Check sheet for the modelled part. Datum: model origin and axes. Units: mm. A direction names the side the tool comes from. Round coordinates to 2 decimals unless told otherwise and drop trailing zeros. Order: outer loops, then holes, each group sorted by start corner. A loop starts at its lowest first (then second) coordinate and runs counter-clockwise, first axis right, second up.
(1) Sectioned sample at C-C, the plane z = -43. Enter the section's corners in (x, y), and give its area (3 significant figures).
(2) Thickness scan on probe 1 along Z at (x, y) = (5, 55); probe 2 along Y at (x, z) = (10.5, -46). Record the ranges inside material, lowest first.
(3) Tool access check on faces 4 (the flat face through (12, 56, -2)), 5 (the flat face through (-5, 119, -28)), 6 (the flat face through (19, 119.1, -12)). Record the directions out of +Z, -Z, +X, -X, +Y, -Y that give a thin tool (end or side, any length) a straight path to the whole face; none if there is none.
(4) Sectioned sample at D-D, the plane z = -51. Enter the section's corners in (x, y).
(5) Depth check by flat-ended pin: pin 1 (0.6 mm diameter, centred on y = 54, z = -1, fed in from -X); pin 2 (16.5 mm diameter, centred on x = 19, z = -21, fed in from -Y). Enter the tip coordinate at first touch or a pass-through.
(6) Sectioned sample at A-A, the plane y = 103. Enter the section's corners in (x, z).
(7) Mould release check, pull along Y, two halves, no side actions. Record for faces 1 (the cylindrical face through (13.56, 8, -0.99)), 2 (the flat face through (11, 63, 0)), 3 (the cylindrical face through (4.68, 10.02, -55.01)): released by +Y, released by -Y, zero draft, split by the parting line, or undercut.
(8) Sectioned sample at B-B, the plane z = -28. Enter the section's corners in (x, y).
```python
from build123d import *

# Parameters (mm, degrees)
SKETCH1_W               = 28
SKETCH1_H               = 124.1
BOSS_EXTRUDE1_DEPTH     = 2
CUT_EXTRUDE2_DEPTH      = 1
CUT_EXTRUDE2_DEPTH_BACK = 2
SKETCH4_R               = 1.25
CUT_EXTRUDE3_DEPTH      = 2
CIRPATTERN1_COUNT       = 5
CIRPATTERN1_ANGLE       = 180
FILLET1_R               = 1.5
SKETCH7_W               = 28
SKETCH7_H               = 124.1
BOSS_EXTRUDE2_DEPTH     = 2
CUT_EXTRUDE4_DEPTH      = 1
CUT_EXTRUDE4_DEPTH_BACK = 2
SKETCH11_R              = 1.25
CUT_EXTRUDE5_DEPTH      = 2
CIRPATTERN2_COUNT       = 5
CIRPATTERN2_ANGLE       = 180
FILLET2_R               = 1.5
SKETCH17_W              = 33
SKETCH17_H              = 52
BOSS_EXTRUDE5_DEPTH     = 15
CUT_EXTRUDE7_REACH      = 126.1
SKETCH18_R              = 3.05
SKETCH19_R              = 1.25
CUT_EXTRUDE8_DEPTH      = 10
SKETCH20_W              = 29.100039055
SKETCH20_H              = 52
CUT_EXTRUDE9_DEPTH      = 5
SKETCH21_W              = 5
SKETCH21_H              = 15
BOSS_EXTRUDE6_DEPTH     = 2
SKETCH22_W              = 52
SKETCH22_H              = 5
CUT_EXTRUDE10_DEPTH     = 2.95
SKETCH23_W              = 52
SKETCH23_H              = 5
CUT_EXTRUDE11_DEPTH     = 2.949960945
CUT_EXTRUDE12_DEPTH     = 3
SKETCH25_R              = 2.5
CUT_EXTRUDE13_DEPTH     = 5


with BuildPart() as part:
    # Sketch1 → Boss-Extrude1 (new body)
    with BuildSketch(Plane.XY):
        with Locations((14, 62.05)):
            Rectangle(SKETCH1_W, SKETCH1_H)
    extrude(amount=-BOSS_EXTRUDE1_DEPTH)

    # Sketch3 → Cut-Extrude2 (cut, two sides)
    with BuildSketch(Plane.XY) as cut_extrude2_sk:
        with BuildLine():
            Line((18.449960945, -261.260932316), (18.449960945, 0))
            Line((18.449960945, 0), (18.449960945, 3))
            ThreePointArc((18.449960945, 3), (13.449960945, 8), (8.449960945, 3))
            Line((8.449960945, 3), (8.449960945, 0))
            Line((8.449960945, 0), (8.449960945, -261.260932316))
            Line((8.449960945, -261.260932316), (8.449960945, -783.782796947))
            Line((8.449960945, -783.782796947), (18.449960945, -783.782796947))
            Line((18.449960945, -783.782796947), (18.449960945, -261.260932316))
        make_face()
    extrude(amount=CUT_EXTRUDE2_DEPTH, mode=Mode.SUBTRACT)
    extrude(cut_extrude2_sk.sketch, amount=-CUT_EXTRUDE2_DEPTH_BACK, mode=Mode.SUBTRACT)

    # Sketch4 → Cut-Extrude3 (cut)
    with BuildSketch(Plane.XY):
        with Locations((2.449960945, 3)):
            Circle(SKETCH4_R)
    cut_extrude3 = extrude(amount=-CUT_EXTRUDE3_DEPTH, mode=Mode.SUBTRACT)

    # CirPattern1: Cut-Extrude3 ×5 about axis
    cirpattern1_axis = Axis((13.449960945, 3, 0), (0, 0, -1))
    for i in range(1, CIRPATTERN1_COUNT):
        add(cut_extrude3.rotate(cirpattern1_axis, i * CIRPATTERN1_ANGLE / (CIRPATTERN1_COUNT - 1)), mode=Mode.SUBTRACT)

    # Fillet1
    fillet1_edges = [part.edges().sort_by_distance(p)[0] for p in [
        (18.449960945, 0, -1),
        (8.449960945, 0, -1),
        (28, 0, -1),
        (0, 0, -1),
    ]]
    fillet(fillet1_edges, radius=FILLET1_R)



with BuildPart() as body_2:
    # Sketch7 → Boss-Extrude2 (new body)
    with BuildSketch(Plane.XY.offset(-56)):
        with Locations((14, 62.05)):
            Rectangle(SKETCH7_W, SKETCH7_H)
    extrude(amount=BOSS_EXTRUDE2_DEPTH)

    # Sketch10 → Cut-Extrude4 (cut, two sides)
    with BuildSketch(Plane(origin=(0, 0, -56), x_dir=(-1, 0, 0), z_dir=(0, 0, -1))) as cut_extrude4_sk:
        with BuildLine():
            Line((-8.449960945, -261.260932316), (-8.449960945, 0))
            Line((-8.449960945, 0), (-8.449960945, 3))
            ThreePointArc((-8.449960945, 3), (-13.449960945, 8), (-18.449960945, 3))
            Line((-18.449960945, 3), (-18.449960945, 0))
            Line((-18.449960945, 0), (-18.449960945, -261.260932316))
            Line((-18.449960945, -261.260932316), (-18.449960945, -783.782796947))
            Line((-18.449960945, -783.782796947), (-8.449960945, -783.782796947))
            Line((-8.449960945, -783.782796947), (-8.449960945, -261.260932316))
        make_face()
    extrude(amount=CUT_EXTRUDE4_DEPTH, mode=Mode.SUBTRACT)
    extrude(cut_extrude4_sk.sketch, amount=-CUT_EXTRUDE4_DEPTH_BACK, mode=Mode.SUBTRACT)

    # Sketch11 → Cut-Extrude5 (cut)
    with BuildSketch(Plane(origin=(0, 0, -56), x_dir=(-1, 0, 0), z_dir=(0, 0, -1))):
        with Locations((-24.449960945, 3)):
            Circle(SKETCH11_R)
    cut_extrude5 = extrude(amount=-CUT_EXTRUDE5_DEPTH, mode=Mode.SUBTRACT)

    # CirPattern2: Cut-Extrude5 ×5 about axis
    cirpattern2_axis = Axis((13.449960945, 3, 0), (0, 0, 1))
    for i in range(1, CIRPATTERN2_COUNT):
        add(cut_extrude5.rotate(cirpattern2_axis, i * CIRPATTERN2_ANGLE / (CIRPATTERN2_COUNT - 1)), mode=Mode.SUBTRACT)

    # Fillet2
    fillet2_edges = [body_2.edges().sort_by_distance(p)[0] for p in [
        (8.449960945, 0, -55),
        (18.449960945, 0, -55),
        (28, 0, -55),
        (0, 0, -55),
    ]]
    fillet(fillet2_edges, radius=FILLET2_R)


with BuildPart() as part_1:
    add(part.part)

    add(body_2.part)  # Boss-Extrude5 merges body 2
    # Sketch17 → Boss-Extrude5 (add)
    with BuildSketch(Plane(origin=(0, 124.1, 0), x_dir=(1, 0, 0), z_dir=(0, 1, 0))):
        with Locations((11.5, 28)):
            Rectangle(SKETCH17_W, SKETCH17_H)
    extrude(amount=-BOSS_EXTRUDE5_DEPTH)

    # Sketch18 → Cut-Extrude7 (cut, up to next)
    with BuildSketch(Plane(origin=(0, 124.1, 0), x_dir=(1, 0, 0), z_dir=(0, 1, 0)), mode=Mode.PRIVATE) as cut_extrude7_sk1:
        with Locations((13.449960945, 28)):
            Circle(SKETCH18_R)
    cut_extrude7_tool1 = extrude(cut_extrude7_sk1.sketch, amount=-CUT_EXTRUDE7_REACH, mode=Mode.PRIVATE) & part_1.part
    add(cut_extrude7_tool1.solids().sort_by_distance((13.449961, 124.1, -28))[0], mode=Mode.SUBTRACT)

    # Sketch19 → Cut-Extrude8 (cut)
    with BuildSketch(Plane(origin=(0, 124.1, 0), x_dir=(1, 0, 0), z_dir=(0, 1, 0))):
        with Locations((0.949960945, 43)):
            Circle(SKETCH19_R)
        with Locations((17.949960945, 43)):
            Circle(SKETCH19_R)
    cut_extrude8 = extrude(amount=-CUT_EXTRUDE8_DEPTH, mode=Mode.SUBTRACT)

    # Mirror9: Cut-Extrude8 across plane
    add(cut_extrude8.mirror(Plane(origin=(0, 0, -28), x_dir=(1, 0, 0), z_dir=(0, 0, -1))), mode=Mode.SUBTRACT)

    # Sketch20 → Cut-Extrude9 (cut)
    with BuildSketch(Plane.XZ.offset(-109.1)):
        with Locations((11.499980473, -28)):
            Rectangle(SKETCH20_W, SKETCH20_H)
    extrude(amount=-CUT_EXTRUDE9_DEPTH, mode=Mode.SUBTRACT)

    # Sketch21 → Boss-Extrude6 (add)
    with BuildSketch(Plane.XY.offset(-2)):
        with Locations((-2.5, 116.6)):
            Rectangle(SKETCH21_W, SKETCH21_H)
    boss_extrude6 = extrude(amount=BOSS_EXTRUDE6_DEPTH)

    # Mirror10: Boss-Extrude6 across plane
    add(boss_extrude6.mirror(Plane(origin=(0, 0, -28), x_dir=(1, 0, 0), z_dir=(0, 0, -1))))

    # Sketch22 → Cut-Extrude10 (cut, through all)
    with BuildSketch(Plane.ZY.offset(-26.05)):
        with Locations((-28, 111.6)):
            Rectangle(SKETCH22_W, SKETCH22_H)
    extrude(amount=-CUT_EXTRUDE10_DEPTH, mode=Mode.SUBTRACT)

    # Sketch23 → Cut-Extrude11 (cut, through all)
    with BuildSketch(Plane(origin=(-3.050039055, 0, 0), x_dir=(0, 0, -1), z_dir=(1, 0, 0))):
        with Locations((28, 111.6)):
            Rectangle(SKETCH23_W, SKETCH23_H)
    extrude(amount=-CUT_EXTRUDE11_DEPTH, mode=Mode.SUBTRACT)

    # Sketch24 → Cut-Extrude12 (cut, through all)
    with BuildSketch(Plane(origin=(0, 0, -2), x_dir=(-1, 0, 0), z_dir=(0, 0, -1))):
        Polygon((0, 109.1), (5, 114.1), (5, 109.1), align=None)
    cut_extrude12 = extrude(amount=-CUT_EXTRUDE12_DEPTH, mode=Mode.SUBTRACT)

    # Mirror11: Cut-Extrude12 across plane
    add(cut_extrude12.mirror(Plane(origin=(0, 0, -28), x_dir=(1, 0, 0), z_dir=(0, 0, -1))), mode=Mode.SUBTRACT)

    # Sketch25 → Cut-Extrude13 (cut)
    with BuildSketch(Plane.XZ.offset(-114.1)):
        with Locations((0.949960945, -43)):
            Circle(SKETCH25_R)
        with Locations((17.949960945, -43)):
            Circle(SKETCH25_R)
    cut_extrude13 = extrude(amount=-CUT_EXTRUDE13_DEPTH, mode=Mode.SUBTRACT)

    # Mirror12: Cut-Extrude13 across plane
    add(cut_extrude13.mirror(Plane(origin=(0, 0, -28), x_dir=(1, 0, 0), z_dir=(0, 0, -1))), mode=Mode.SUBTRACT)


solid = part_1.part
```
Derived:
1. outline: (-5, 114.1) - (-1.55, 114.1) - (-1.55, 119.1) - (-0.3, 119.1) - (-0.3, 124.1) - (-5, 124.1) - close; (2.2, 119.1) - (3.45, 119.1) - (3.45, 114.1) - (15.45, 114.1) - (15.45, 119.1) - (16.7, 119.1) - (16.7, 124.1) - (2.2, 124.1) - close; (19.2, 119.1) - (20.45, 119.1) - (20.45, 114.1) - (28, 114.1) - (28, 124.1) - (19.2, 124.1) - close
1. area: 255 mm2
2. probe 1: z = -56 to -54, -2 to 0
2. probe 2: y = 114.1 to 124.1
3. face 4: +X, -X, -Y
3. face 5: +Z, -Z, -X, +Y, -Y
3. face 6: -Y
4. outline: (-5, 114.1) - (28, 114.1) - (28, 124.1) - (-5, 124.1) - close
5. pin 1: stops at x = 0
5. pin 2: stops at y = 114.1
6. outline: (0, -56) - (28, -56) - (28, -54) - (0, -54) - close; (0, -2) - (28, -2) - (28, 0) - (0, 0) - close
7. face 1: released by -Y
7. face 2: zero draft
7. face 3: undercut
8. outline: (-5, 114.1) - (10.4, 114.1) - (10.4, 124.1) - (-5, 124.1) - close; (16.5, 114.1) - (28, 114.1) - (28, 124.1) - (16.5, 124.1) - close
